The listing builds one solid part. Answer for the finished solid, in the listing's coordinates (mm). Face numbers are marked on the shaded views. Coordinates: 2 decimals unless noted, no trailing zeros. Order: outer loops, then holes, each group sorted by start corner. A loop starts at its lowest first (then second) coordinate and runs counter-clockwise, first axis right, second up.
from build123d import *

# Parameters (mm, degrees)
BOSS_EXTRU_1_DEPTH = 45


with BuildPart() as part:
    # Esquisse1 → Boss.-Extru.1 (new body)
    with BuildSketch(Plane.XY):
        with BuildLine():
            Line((-46, 10.057417596), (-46, -10.057417596))
            ThreePointArc((-46, -10.057417596), (-45.795643546, -10.303215616), (-45.516666667, -10.147170343))
            ThreePointArc((-45.516666667, -10.147170343), (-37.426337153, -5.621857418), (-31.5, -12.75))
            ThreePointArc((-31.5, -12.75), (-31, -13.25), (-30.5, -12.75))
            ThreePointArc((-30.5, -12.75), (-23.25, -5.5), (-16, -12.75))
            ThreePointArc((-16, -12.75), (-15.5, -13.25), (-15, -12.75))
            ThreePointArc((-15, -12.75), (-7.75, -5.5), (-0.5, -12.75))
            ThreePointArc((-0.5, -12.75), (0, -13.25), (0.5, -12.75))
            ThreePointArc((0.5, -12.75), (7.75, -5.5), (15, -12.75))
            ThreePointArc((15, -12.75), (15.5, -13.25), (16, -12.75))
            ThreePointArc((16, -12.75), (23.25, -5.5), (30.5, -12.75))
            ThreePointArc((30.5, -12.75), (31, -13.25), (31.5, -12.75))
            ThreePointArc((31.5, -12.75), (37.426337153, -5.621857418), (45.516666667, -10.147170343))
            ThreePointArc((45.516666667, -10.147170343), (45.795643546, -10.303215616), (46, -10.057417596))
            Line((46, -10.057417596), (46, 10.057417596))
            ThreePointArc((46, 10.057417596), (45.795643546, 10.303215616), (45.516666667, 10.147170343))
            ThreePointArc((45.516666667, 10.147170343), (37.426337153, 5.621857418), (31.5, 12.75))
            ThreePointArc((31.5, 12.75), (31, 13.25), (30.5, 12.75))
            ThreePointArc((30.5, 12.75), (23.25, 5.5), (16, 12.75))
            ThreePointArc((16, 12.75), (15.5, 13.25), (15, 12.75))
            ThreePointArc((15, 12.75), (7.75, 5.5), (0.5, 12.75))
            ThreePointArc((0.5, 12.75), (0, 13.25), (-0.5, 12.75))
            ThreePointArc((-0.5, 12.75), (-7.75, 5.5), (-15, 12.75))
            ThreePointArc((-15, 12.75), (-15.5, 13.25), (-16, 12.75))
            ThreePointArc((-16, 12.75), (-23.25, 5.5), (-30.5, 12.75))
            ThreePointArc((-30.5, 12.75), (-31, 13.25), (-31.5, 12.75))
            ThreePointArc((-31.5, 12.75), (-37.426337153, 5.621857418), (-45.516666667, 10.147170343))
            ThreePointArc((-45.516666667, 10.147170343), (-45.795643546, 10.303215616), (-46, 10.057417596))
        make_face()
    extrude(amount=BOSS_EXTRU_1_DEPTH)


solid = part.part
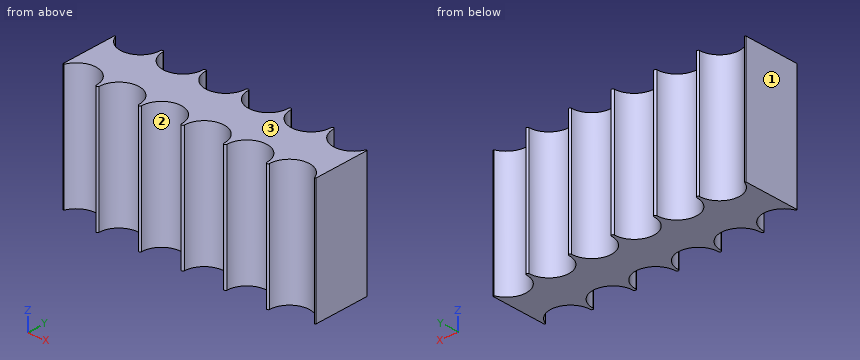
(1) Find section C-C on x = -23.25. Determine the outline of the cut face in (y, z).
(2) Find the intervals of material crossed by probe 1 along X at (y, z) = (12.25, 42.5); probe 2 along X at (y, z) = (-11.25, 6); probe 3 along Y at (x, z) = (-23, 35.5), in increasing order.
(3) Given pin 1 Ø1 at (x, z) = (-29, 29.5) entering from -Y; pin 2 Ø6 at (x, z) = (-8, 26.5) entering from -Y; pin 3 Ø3 at (x, z) = (8, 7.5) entering from +Y, each flat-ended and moving along its own axis, determine where each tip first touches the part or whether it passes through.
(4) Find section D-D on y = -7. Determine the outline of the cut face in (x, z).
(5) Find section A-A on y = 7.5. Determine the outline of the cut face in (x, z), then the cut area to 3 significant figures.
(6) The mould has two halves that part along X. Classify the marked faces 1, 2 and 3: pulls with the +X half, pulls with the -X half, needs draft (parallel to the pull), parting line crosses it, or undercut.
(7) Find section B-B on z = 5.5. Determine the outline of the cut face in (x, y), then the cut area to 3 significant figures.
Resolved:
1. outline: (-5.5, 0) - (5.5, 0) - (5.5, 45) - (-5.5, 45) - close
2. probe 1: x = -31.52 to -30.48, -16.02 to -14.98, -0.52 to 0.52, 14.98 to 16.02, 30.48 to 31.52
2. probe 2: x = -31.66 to -30.34, -16.16 to -14.84, -0.66 to 0.66, 14.84 to 16.16, 30.34 to 31.66
2. probe 3: y = -5.5 to 5.5
3. pin 1: stops at y = -9.08
3. pin 2: stops at y = -6.27
3. pin 3: stops at y = 5.71
4. outline: (-46, 0) - (-43.17, 0) - (-43.17, 45) - (-46, 45) - close; (-34.33, 0) - (-27.67, 0) - (-27.67, 45) - (-34.33, 45) - close; (-18.83, 0) - (-12.17, 0) - (-12.17, 45) - (-18.83, 45) - close; (-3.33, 0) - (3.33, 0) - (3.33, 45) - (-3.33, 45) - close; (12.17, 0) - (18.83, 0) - (18.83, 45) - (12.17, 45) - close; (27.67, 0) - (34.33, 0) - (34.33, 45) - (27.67, 45) - close; (43.17, 0) - (46, 0) - (46, 45) - (43.17, 45) - close
5. outline: (-46, 0) - (-43.75, 0) - (-43.75, 45) - (-46, 45) - close; (-33.75, 0) - (-28.25, 0) - (-28.25, 45) - (-33.75, 45) - close; (-18.25, 0) - (-12.75, 0) - (-12.75, 45) - (-18.25, 45) - close; (-2.75, 0) - (2.75, 0) - (2.75, 45) - (-2.75, 45) - close; (12.75, 0) - (18.25, 0) - (18.25, 45) - (12.75, 45) - close; (28.25, 0) - (33.75, 0) - (33.75, 45) - (28.25, 45) - close; (43.75, 0) - (46, 0) - (46, 45) - (43.75, 45) - close
5. area: 1,440 mm2
6. face 1: pulls with the -X half
6. face 2: undercut
6. face 3: needs draft
7. outline: (-46, -10.06) arc R0.25 ccw to (-45.52, -10.15) arc R7.25 cw to (-31.5, -12.75) arc R0.5 ccw to (-30.5, -12.75) arc R7.25 cw to (-16, -12.75) arc R0.5 ccw to (-15, -12.75) arc R7.25 cw to (-0.5, -12.75) arc R0.5 ccw to (0.5, -12.75) arc R7.25 cw to (15, -12.75) arc R0.5 ccw to (16, -12.75) arc R7.25 cw to (30.5, -12.75) arc R0.5 ccw to (31.5, -12.75) arc R7.25 cw to (45.52, -10.15) arc R0.25 ccw to (46, -10.06) - (46, 10.06) arc R0.25 ccw to (45.52, 10.15) arc R7.25 cw to (31.5, 12.75) arc R0.5 ccw to (30.5, 12.75) arc R7.25 cw to (16, 12.75) arc R0.5 ccw to (15, 12.75) arc R7.25 cw to (0.5, 12.75) arc R0.5 ccw to (-0.5, 12.75) arc R7.25 cw to (-15, 12.75) arc R0.5 ccw to (-16, 12.75) arc R7.25 cw to (-30.5, 12.75) arc R0.5 ccw to (-31.5, 12.75) arc R7.25 cw to (-45.52, 10.15) arc R0.25 ccw to (-46, 10.06) - close
7. area: 1,360 mm2
